from build123d import *

# Parameters (mm, degrees)
SKETCH_W        = 1800
SKETCH_H        = 800
PAD_DEPTH       = 20
SKETCH001_W     = 580
SKETCH001_H     = 90
POCKET_DEPTH    = 20
SKETCH002_W     = 120
SKETCH002_H     = 120
POCKET001_DEPTH = 20


with BuildPart() as part:
    # Sketch → Pad (new body)
    with BuildSketch(Plane.XY):
        Rectangle(SKETCH_W, SKETCH_H)
    extrude(amount=PAD_DEPTH)

    # Sketch001 (on Face6 of Pad) → Pocket (cut)
    with BuildSketch(Plane.XY.offset(20)):
        with Locations((210, -355)):
            Rectangle(SKETCH001_W, SKETCH001_H)
        with Locations((210, 355)):
            Rectangle(SKETCH001_W, SKETCH001_H)
    extrude(amount=-POCKET_DEPTH, mode=Mode.SUBTRACT)

    # Sketch002 (on Face4 of Pocket) → Pocket001 (cut)
    with BuildSketch(Plane(origin=(0, 0, 0), x_dir=(1, 0, 0), z_dir=(0, 0, -1))):
        with Locations((-92.5, 240)):
            Rectangle(SKETCH002_W, SKETCH002_H)
        with Locations((512.5, 240)):
            Rectangle(SKETCH002_W, SKETCH002_H)
        with Locations((-92.5, -240)):
            Rectangle(SKETCH002_W, SKETCH002_H)
        with Locations((512.5, -240)):
            Rectangle(SKETCH002_W, SKETCH002_H)
    extrude(amount=-POCKET001_DEPTH, mode=Mode.SUBTRACT)


solid = part.part
Verification items for the finished model (mm, model axes). Coordinates: 2 decimals unless noted, no trailing zeros. Loops run counter-clockwise (first coordinate to the right, second up) from the corner with the lowest first, then second, coordinate; pieces in that order, holes last. Notation, with made-up numbers: (76, 54.5) -> (122, 54.5) arc R19 ccw to (122, 71.5) -> close; hole circle Ø11 at (87, -36). An arc over 180 degrees is marked (long way). Answer as CSV lines item,"result".
1) Thickness scan on L1, parallel to X at y = 225, z = 4.75; L2, parallel to X at y = 366, z = 12.25; L3, parallel to Y at x = 313.5, z = 6. Record the ranges inside material, lowest first. Write a range as from..to.
Found:
L1,"x = -900..-152.5, -32.5..452.5, 572.5..900"
L2,"x = -900..-80, 500..900"
L3,"y = -310..310"
2) Cross-section at B-B, the plane x = 209. Record the cut outline in (y, z), then the cut area to 3 significant figures.
Found:
outline,"(-310, 0) -> (310, 0) -> (310, 20) -> (-310, 20) -> close"
area,"12,400 mm2"
3) Cross-section at A-A, the plane z = 7. Record the cut outline in (x, y).
Found:
outline,"(-900, -400) -> (-80, -400) -> (-80, -310) -> (500, -310) -> (500, -400) -> (900, -400) -> (900, 400) -> (500, 400) -> (500, 310) -> (-80, 310) -> (-80, 400) -> (-900, 400) -> close; hole (-152.5, -300) -> (-32.5, -300) -> (-32.5, -180) -> (-152.5, -180) -> close; hole (-152.5, 180) -> (-32.5, 180) -> (-32.5, 300) -> (-152.5, 300) -> close; hole (452.5, -300) -> (572.5, -300) -> (572.5, -180) -> (452.5, -180) -> close; hole (452.5, 180) -> (572.5, 180) -> (572.5, 300) -> (452.5, 300) -> close"
4) Depth check by flat-ended pin: pin 1 (1.5 mm diameter, centred on x = -702.5, y = 116.5, fed in from -Z); pin 2 (6 mm diameter, centred on x = -76, z = 9, fed in from +Y); pin 3 (6 mm diameter, centred on x = 142.5, z = 7.5, fed in from -Y). Enter the tip coordinate at first touch or a pass-through.
Found:
pin 1,"stops at z = 0"
pin 2,"stops at y = 310"
pin 3,"stops at y = -310"
